Verification items for the finished model (mm, model axes). Give positions to 0.01 mm unless a question says otherwise; leave off trailing zeros. Write each loop counter-clockwise with the first axis right and the second up, starting at its lowest first coordinate (ties: lowest second). Pieces come first, ordered by that corner, then holes.
Autodesk Inventor part; units mm, degrees
ref_plane "YZ Plane" through (0, 0, 0) normal (1, 0, 0) x (0, 1, 0)
ref_plane "XZ Plane" through (0, 0, 0) normal (0, 1, 0) x (-1, 0, 0)
ref_plane "XY Plane" through (0, 0, 0) normal (0, 0, 1) x (1, 0, 0)
sketch "Sketch1" plane through (0, 0, 0) normal (0, 0, 1) x (1, 0, 0)
  line L0 (-145, -145) -> (145, -145)
  line L1 (145, -145) -> (145, 145)
  line L2 (145, 145) -> (-145, 145)
  line L3 (-145, 145) -> (-145, -145)
  line L4 (-145, -145) -> (145, 145) construction
  line L5 (145, -145) -> (-145, 145) construction
  point P0 (0, 0)
  dimension "d0" = 290
  dimension "d1" = 290
extrude "Extrusion1" add sketch "Sketch1" along normal blind 5
sketch "Sketch2" plane through (0, 0, 5) normal (0, 0, 1) x (1, 0, 0)
  line L0 (-137.5, -137.5) -> (137.5, -137.5) construction
  line L1 (137.5, -137.5) -> (137.5, 137.5) construction
  line L2 (137.5, 137.5) -> (-137.5, 137.5) construction
  line L3 (-137.5, 137.5) -> (-137.5, -137.5) construction
  line L4 (-137.5, -137.5) -> (137.5, 137.5) construction
  line L5 (137.5, -137.5) -> (-137.5, 137.5) construction
  point P0 (0, 0)
  dimension "d4" = 275
  dimension "d5" = 275
hole "Hole1" at (-137.5, 137.5, 5) at (137.5, 137.5, 5) at (137.5, -137.5, 5) at (-137.5, -137.5, 5) direction (0, 0, -1) diameter 5.5 depth 8 tip angle 118
sketch "Sketch3" plane through (0, 0, 5) normal (0, 0, 1) x (1, 0, 0)
  line L0 (-123, 112.5) -> (12, 112.5) construction
  line L1 (12, 112.5) -> (12, -112.5) construction
  line L2 (12, -112.5) -> (-123, -112.5) construction
  line L3 (-123, -112.5) -> (-123, 112.5) construction
  line L4 (-145, 145) -> (-145, -145)
  line L5 (145, -145) -> (145, 145)
  point P0 (0, 0)
  point P1 (12, 0)
  dimension "d13" = 135
  dimension "d34" = 225
  dimension "d35" = 22
hole "Hole2" at (-123, 112.5, 5) at (12, 112.5, 5) at (12, -112.5, 5) at (-123, -112.5, 5) direction (0, 0, -1) diameter 3.4 depth 8 tip angle 118
sketch "Sketch4" plane through (0, 0, 5) normal (0, 0, 1) x (1, 0, 0)
  line L0 (-140, 120) -> (-135, 120)
  line L1 (-135, 120) -> (-135, -120)
  line L2 (-135, -120) -> (-140, -120)
  line L3 (-140, -120) -> (-140, 120)
  line L4 (-120, -140) -> (120, -140)
  line L5 (120, -140) -> (120, -135)
  line L6 (120, -135) -> (-120, -135)
  line L7 (-120, -135) -> (-120, -140)
  line L8 (140, -120) -> (135, -120)
  line L9 (135, -120) -> (135, 120)
  line L10 (135, 120) -> (140, 120)
  line L11 (140, 120) -> (140, -120)
  line L12 (120, 140) -> (-120, 140)
  line L13 (-120, 140) -> (-120, 135)
  line L14 (-120, 135) -> (120, 135)
  line L15 (120, 135) -> (120, 140)
  line L16 (-145, 145) -> (-145, -145)
  line L17 (145, 145) -> (-145, 145)
  line L18 (145, -145) -> (145, 145)
  line L19 (-145, -145) -> (145, -145)
  point P0 (0, 0)
  point P1 (0, 135)
  point P2 (0, -135)
  point P3 (-135, 0)
  point P4 (135, 0)
  dimension "d21" = 240
  dimension "d22" = 240
  dimension "d23" = 5
  dimension "d24" = 5
  dimension "d25" = 5
  dimension "d26" = 5
  dimension "d27" = 5
  dimension "d28" = 5
  dimension "d29" = 5
  dimension "d30" = 5
extrude "Extrusion2" cut sketch "Sketch4" against normal blind 10 contours L0 L1 L2 L3 | L7 L6 L5 L4 | L8 L9 L10 L11 | L15 L14 L13 L12
fillet "Fillet1" radius 6 4 edges at (-145, -145, 2.5) (145, -145, 2.5) (145, 145, 2.5) (-145, 145, 2.5)
sketch "Sketch6" plane through (0, 0, 5) normal (0, 0, 1) x (1, 0, 0)
  line L0 (135, -120) -> (135, 120) construction
  line L1 (21.5, 12.5) -> (26.5, 12.5)
  line L2 (26.5, 12.5) -> (26.5, 50)
  line L3 (26.5, 50) -> (21.5, 50)
  line L4 (21.5, 50) -> (21.5, 12.5)
  line L5 (21.5, -12.5) -> (26.5, -12.5)
  line L6 (26.5, -12.5) -> (26.5, -50)
  line L7 (26.5, -50) -> (21.5, -50)
  line L8 (21.5, -50) -> (21.5, -12.5)
  line L9 (90, -64) -> (85, -64)
  line L10 (85, -64) -> (85, -26.5)
  line L11 (85, -26.5) -> (90, -26.5)
  line L12 (90, -26.5) -> (90, -64)
  line L13 (90, -1.5) -> (85, -1.5)
  line L14 (85, -1.5) -> (85, 36)
  line L15 (85, 36) -> (90, 36)
  line L16 (90, 36) -> (90, -1.5)
  line L17 (21.5, -12.5) -> (21.5, 12.5) construction
  point P0 (0, 0)
  point P1 (21.5, 0)
  dimension "d95" = 5
  dimension "d96" = 37.5
  dimension "d97" = 37.5
  dimension "d98" = 5
  dimension "d99" = 25
  dimension "d100" = 21.5
  dimension "d101" = 37.5
  dimension "d102" = 5
  dimension "d103" = 37.5
  dimension "d104" = 25
  dimension "d105" = 58.5
  dimension "d113" = 14
extrude "Extrusion3" cut sketch "Sketch6" against normal through all
sketch "Sketch7" plane through (0, 0, 5) normal (0, 0, 1) x (1, 0, 0)
  line L0 (21.5, 12.5) -> (21.5, 50)
  line L1 (26.5, 12.5) -> (21.5, 12.5)
  line L2 (85, -1.5) -> (85, 36)
  line L3 (90, -1.5) -> (85, -1.5)
  line L4 (85, -26.5) -> (90, -26.5)
  line L5 (21.5, -12.5) -> (26.5, -12.5)
  point P0 (0, 0)
  point P1 (24, 0)
  point P2 (87.5, -14)
  dimension "d107" = 2.5
  dimension "d108" = 2.5
  dimension "d109" = 25
  dimension "d110" = 12.5
  dimension "d111" = 25
  dimension "d112" = 12.5
hole "Hole3" at (24, 0, 5) at (87.5, -14, 5) direction (0, 0, -1) diameter 4.5 depth 8 tip angle 118
sketch "Sketch11" plane through (0, 0, 5) normal (0, 0, 1) x (1, 0, 0)
  circle A0 centre (12, 112.5) radius 1.7
  circle A1 centre (-123, 112.5) radius 1.7
  circle A2 centre (-123, -112.5) radius 1.7
  circle A3 centre (12, -112.5) radius 1.7
  line L0 (12, 112.5) -> (-123, 112.5) construction
  line L1 (-123, 112.5) -> (-123, -112.5) construction
  line L2 (-123, -112.5) -> (12, -112.5) construction
  line L3 (12, -112.5) -> (12, 112.5) construction
  line L4 (-5.5, 0) -> (-105.5, 0) construction
  line L5 (-5.5, 2.5) -> (-105.5, 2.5)
  line L6 (-105.5, -2.5) -> (-5.5, -2.5)
  arc A4 (-5.5, -2.5) -> (-5.5, 2.5) centre (-5.5, 0) ccw
  arc A5 (-105.5, 2.5) -> (-105.5, -2.5) centre (-105.5, 0) ccw
  line L7 (-5.5, 40) -> (-105.5, 40) construction
  line L8 (-5.5, 42.5) -> (-105.5, 42.5)
  line L9 (-105.5, 37.5) -> (-5.5, 37.5)
  arc A6 (-5.5, 37.5) -> (-5.5, 42.5) centre (-5.5, 40) ccw
  arc A7 (-105.5, 42.5) -> (-105.5, 37.5) centre (-105.5, 40) ccw
  line L10 (-5.5, 80) -> (-105.5, 80) construction
  line L11 (-5.5, 82.5) -> (-105.5, 82.5)
  line L12 (-105.5, 77.5) -> (-5.5, 77.5)
  arc A8 (-5.5, 77.5) -> (-5.5, 82.5) centre (-5.5, 80) ccw
  arc A9 (-105.5, 82.5) -> (-105.5, 77.5) centre (-105.5, 80) ccw
  line L13 (-5.5, -37.5) -> (-105.5, -37.5)
  line L14 (-5.5, -40) -> (-105.5, -40) construction
  line L15 (-105.5, -42.5) -> (-5.5, -42.5)
  arc A10 (-5.5, -42.5) -> (-5.5, -37.5) centre (-5.5, -40) ccw
  arc A11 (-105.5, -37.5) -> (-105.5, -42.5) centre (-105.5, -40) ccw
  line L16 (-5.5, -77.5) -> (-105.5, -77.5)
  line L17 (-5.5, -80) -> (-105.5, -80) construction
  line L18 (-105.5, -82.5) -> (-5.5, -82.5)
  arc A12 (-5.5, -82.5) -> (-5.5, -77.5) centre (-5.5, -80) ccw
  arc A13 (-105.5, -77.5) -> (-105.5, -82.5) centre (-105.5, -80) ccw
  point P0 (0, 0)
  point P1 (-55.5, 0)
  point P2 (-55.5, 40)
  point P3 (-55.5, 80)
  point P4 (-55.5, -40)
  point P5 (-55.5, -80)
  dimension "d114" = 5
  dimension "d115" = 100
  dimension "d116" = 135
  dimension "d117" = 17.5
  dimension "d120" = 40
  dimension "d127" = 40
extrude "Extrusion4" cut sketch "Sketch11" against normal blind 10 contours A4 L6 A5 L5 | A6 L9 A7 L8 | A8 L12 A9 L11 | A10 L15 A11 L13 | A12 L18 A13 L16
equation "\"d117\" = -0.5 * d115 + 0.5 * d116"
properties part number "bottom" material "Polycarbonate, Clear"
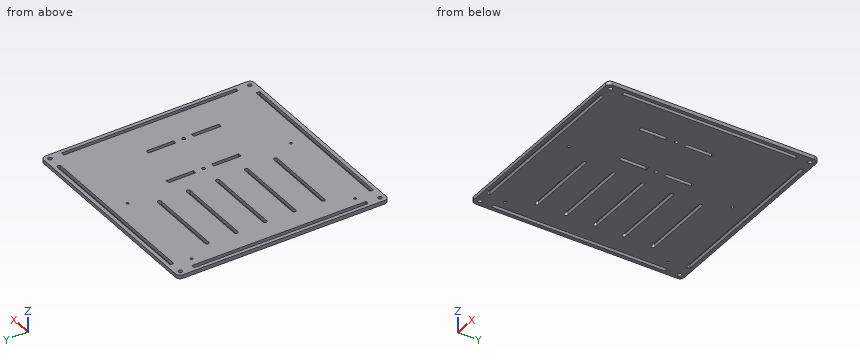
Item 1: Scan lines: line 1 along X through (y, z) = (112.5, 1); line 2 along Y through (x, z) = (104, 3.2); line 3 along Y through (x, z) = (-137.5, 3.3). Record each from-to range of solid material in increasing order.
Answer key:
line 1: x = -145 to -140, -135 to -124.7, -121.3 to 10.3, 13.7 to 135, 140 to 145
line 2: y = -145 to -140, -135 to 135, 140 to 145
line 3: y = -145 to -140.25, -134.75 to -120, 120 to 134.75, 140.25 to 145
Item 2: Depth check by flat-ended pin: pin 1 (1.5 mm diameter, centred on x = 61, y = -96.5, fed in from -Z); pin 2 (3 mm diameter, centred on x = 12, y = -112.5, fed in from +Z). Enter the tip coordinate at first touch or a pass-through.
Answer key:
pin 1: stops at z = 0
pin 2: passes through
Item 3: Sectioned sample at A-A on x = 76. Record the cut outline in (y, z).
Answer key:
outline: (-145, 0) - (-140, 0) - (-140, 5) - (-145, 5) - close; (-135, 0) - (135, 0) - (135, 5) - (-135, 5) - close; (140, 0) - (145, 0) - (145, 5) - (140, 5) - close
Item 4: Sectioned sample at C-C on x = -25.5. State how many separate pieces and enclosed holes the cut face has, then the cut area to 4 significant figures.
Answer key:
separate pieces: 8
enclosed holes: 0
area: 1,275 mm2
